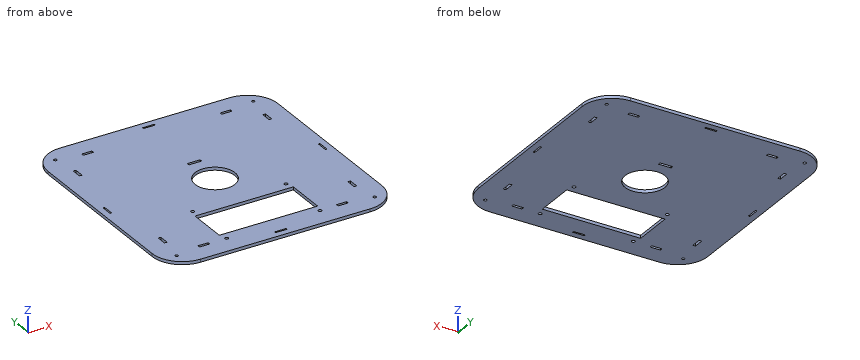
```python
from build123d import *

# Parameters (mm, degrees)
CROQUIS1_R              = 1.5
CROQUIS1_R_2            = 1.75
CROQUIS1_R_3            = 20
CROQUIS1_W              = 98.5
CROQUIS1_H              = 39.8
CROQUIS1_W_2            = 10.2
CROQUIS1_H_2            = 2.6
CROQUIS1_W_3            = 2.6
CROQUIS1_H_3            = 10.2
CROQUIS1_W_4            = 1.6
CROQUIS1_H_4            = 11.6
CROQUIS1_W_5            = 12.8
CROQUIS1_H_5            = 2.62
CROQUIS1_W_6            = 11.6
CROQUIS1_H_6            = 1.6
SALIENTE_EXTRUIR1_DEPTH = 3


with BuildPart() as part:
    # Croquis1 → Saliente-Extruir1 (new body)
    with BuildSketch(Plane.XY):
        with BuildLine():
            Line((85, -115), (-85, -115))
            ThreePointArc((-85, -115), (-106.213203436, -106.213203436), (-115, -85))
            Line((-115, -85), (-115, 85))
            ThreePointArc((-115, 85), (-106.213203436, 106.213203436), (-85, 115))
            Line((-85, 115), (85, 115))
            ThreePointArc((85, 115), (106.213203436, 106.213203436), (115, 85))
            Line((115, 85), (115, -85))
            ThreePointArc((115, -85), (106.213203436, -106.213203436), (85, -115))
        make_face()
        with Locations((-99.142135624, 99.142135624)):
            Circle(CROQUIS1_R, mode=Mode.SUBTRACT)
        with Locations((-99.142135624, -99.142135624)):
            Circle(CROQUIS1_R, mode=Mode.SUBTRACT)
        with Locations((99.142135624, 99.142135624)):
            Circle(CROQUIS1_R, mode=Mode.SUBTRACT)
        with Locations((99.142135624, -99.142135624)):
            Circle(CROQUIS1_R, mode=Mode.SUBTRACT)
        with Locations((46.7, -39.75)):
            Circle(CROQUIS1_R_2, mode=Mode.SUBTRACT)
        with Locations((-46.7, -39.75)):
            Circle(CROQUIS1_R_2, mode=Mode.SUBTRACT)
        with Locations((46.7, -95.25)):
            Circle(CROQUIS1_R_2, mode=Mode.SUBTRACT)
        with Locations((-46.7, -95.25)):
            Circle(CROQUIS1_R_2, mode=Mode.SUBTRACT)
        Circle(CROQUIS1_R_3, mode=Mode.SUBTRACT)
        with Locations((0, -67.5)):
            Rectangle(CROQUIS1_W, CROQUIS1_H, mode=Mode.SUBTRACT)
        with Locations((69.375, 95)):
            Rectangle(CROQUIS1_W_2, CROQUIS1_H_2, mode=Mode.SUBTRACT)
        with Locations((69.375, -95)):
            Rectangle(CROQUIS1_W_2, CROQUIS1_H_2, mode=Mode.SUBTRACT)
        with Locations((-69.375, -95)):
            Rectangle(CROQUIS1_W_2, CROQUIS1_H_2, mode=Mode.SUBTRACT)
        with Locations((-69.375, 95)):
            Rectangle(CROQUIS1_W_2, CROQUIS1_H_2, mode=Mode.SUBTRACT)
        with Locations((-95, -69.375)):
            Rectangle(CROQUIS1_W_3, CROQUIS1_H_3, mode=Mode.SUBTRACT)
        with Locations((-95, 69.375)):
            Rectangle(CROQUIS1_W_3, CROQUIS1_H_3, mode=Mode.SUBTRACT)
        with Locations((95, -69.375)):
            Rectangle(CROQUIS1_W_3, CROQUIS1_H_3, mode=Mode.SUBTRACT)
        with Locations((95, 69.375)):
            Rectangle(CROQUIS1_W_3, CROQUIS1_H_3, mode=Mode.SUBTRACT)
        with Locations((107.843441478, 0)):
            Rectangle(CROQUIS1_W_4, CROQUIS1_H_4, mode=Mode.SUBTRACT)
        with Locations((0, 33.445401683)):
            Rectangle(CROQUIS1_W_5, CROQUIS1_H_5, mode=Mode.SUBTRACT)
        with Locations((-107.843441478, 0)):
            Rectangle(CROQUIS1_W_4, CROQUIS1_H_4, mode=Mode.SUBTRACT)
        with Locations((0, 107.843441478)):
            Rectangle(CROQUIS1_W_6, CROQUIS1_H_6, mode=Mode.SUBTRACT)
        with Locations((0, -107.843441478)):
            Rectangle(CROQUIS1_W_6, CROQUIS1_H_6, mode=Mode.SUBTRACT)
    extrude(amount=SALIENTE_EXTRUIR1_DEPTH)


solid = part.part
```
Work out the finished part from the listing and answer in its coordinate system (mm). Give positions to 0.01 mm unless a question says otherwise; leave off trailing zeros. Loops run counter-clockwise (first coordinate to the right, second up) from the corner with the lowest first, then second, coordinate; pieces in that order, holes last. Notation, with made-up numbers: M -25.75,34.25 L -21.75,34.25 A26 cw -21.75,69.25 Z; hole C 21.5,-1 d4. An arc over 180 degrees is marked long. One line per item, written item: value. Start each with the question number.
1. Find section B-B (x = 0). Give the vertices of the cut face in (y, z), and give its area (3 significant figures).
2. Find the intervals of material crossed by probe 1 along Y at (x, z) = (-46.7, 1.05); probe 2 along Y at (x, z) = (-69, 2.2), in increasing order.
3. Find section A-A (y = 0). Give the vertices of the cut face in (x, z).
4. Find section D-D (z = 1.1). State how many separate pieces and enclosed holes the cut face has, and give its area (3 significant figures).
5. Find section C-C (y = -55.5). Give the vertices of the cut face in (x, z).
6. Each of these flat-tipped pins is pushed along its axis until it touches: P1, Ø1.3, axis at x = 108, z = 1.5, coming from the -Y side; P2, Ø1.3, axis at x = -108, z = 2, coming from the +Y side; P3, Ø0.8, axis at y = -95.5, z = 2, coming from the +X side. Where does it stop, or does it pass through?
Reported:
1. outline: M -115,0 L -108.64,0 L -108.64,3 L -115,3 Z; M -107.04,0 L -87.4,0 L -87.4,3 L -107.04,3 Z; M -47.6,0 L -20,0 L -20,3 L -47.6,3 Z; M 20,0 L 32.14,0 L 32.14,3 L 20,3 Z; M 34.76,0 L 107.04,0 L 107.04,3 L 34.76,3 Z; M 108.64,0 L 115,0 L 115,3 L 108.64,3 Z
1. area: 433 mm²
2. probe 1: y = -115 to -97, -93.5 to -87.4, -47.6 to -41.5, -38 to 115
2. probe 2: y = -115 to -96.3, -93.7 to 93.7, 96.3 to 115
3. outline: M -115,0 L -108.64,0 L -108.64,3 L -115,3 Z; M -107.04,0 L -20,0 L -20,3 L -107.04,3 Z; M 20,0 L 107.04,0 L 107.04,3 L 20,3 Z; M 108.64,0 L 115,0 L 115,3 L 108.64,3 Z
4. separate pieces: 1
4. enclosed holes: 23
4. area: 46,600 mm²
5. outline: M -115,0 L -49.25,0 L -49.25,3 L -115,3 Z; M 49.25,0 L 115,0 L 115,3 L 49.25,3 Z
6. P1: stops at y = -105.01
6. P2: stops at y = 105.01
6. P3: stops at x = 113.25
